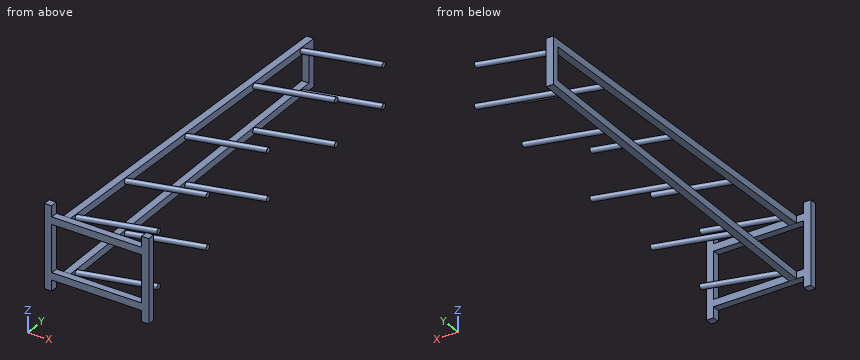
```python
from build123d import *

# Parameters (mm, degrees)
SKETCH1_W           = 25.4
SKETCH1_H           = 25.4
BOSS_EXTRUDE1_DEPTH = 292.1
SKETCH2_W           = 25.4
SKETCH2_H           = 25.4
BOSS_EXTRUDE2_DEPTH = 317.5
BOSS_EXTRUDE3_DEPTH = 25.4
SKETCH4_R           = 9.525
BOSS_EXTRUDE5_DEPTH = 254


with BuildPart() as part:
    # Sketch1 → Boss-Extrude1 (new body)
    with BuildSketch(Plane.XY):
        with Locations((12.7, 12.7)):
            Rectangle(SKETCH1_W, SKETCH1_H)
    boss_extrude1 = extrude(amount=BOSS_EXTRUDE1_DEPTH)

    # Sketch2 → Boss-Extrude2 (add)
    with BuildSketch(Plane(origin=(25.4, 0, 0), x_dir=(0, 0, -1), z_dir=(1, 0, 0))):
        with Locations((-241.3, 12.7)):
            Rectangle(SKETCH2_W, SKETCH2_H)
        with Locations((-50.8, 12.7)):
            Rectangle(SKETCH2_W, SKETCH2_H)
    extrude(amount=BOSS_EXTRUDE2_DEPTH)

    # Mirror1: Boss-Extrude1 across plane
    add(boss_extrude1.mirror(Plane(origin=(184.15, 0, 0), x_dir=(0, 0, 1), z_dir=(1, 0, 0))))

    # Sketch3 → Boss-Extrude3 (add)
    with BuildSketch(Plane.ZY.offset(-50.8)):
        Polygon((38.1, 25.4), (63.5, 1320.8), (88.904882268, 1320.8), (203.195117732, 1320.8), (228.6, 1320.8), (254, 25.4), (228.595117732, 25.4), (203.693156948, 1295.4), (88.406843052, 1295.4), (63.504882268, 25.4), align=None)
    extrude(amount=-BOSS_EXTRUDE3_DEPTH)

    # Sketch4 → Boss-Extrude5 (add, along a direction that is not the sketch's normal)
    with BuildSketch(Plane(origin=(76.2, 0, 0), x_dir=(0, 0, -1), z_dir=(1, 0, 0))):
        with Locations((-240.674544157, 57.298247998)):
            Circle(SKETCH4_R)
        with Locations((-235.530825048, 319.62792253)):
            Circle(SKETCH4_R)
        with Locations((-229.210655655, 641.956561596)):
            Circle(SKETCH4_R)
        with Locations((-217.142014813, 1257.457244551)):
            Circle(SKETCH4_R)
        with Locations((-222.108994477, 1004.141281654)):
            Circle(SKETCH4_R)
    boss_extrude5 = extrude(amount=BOSS_EXTRUDE5_DEPTH, dir=(0.9659258262890673, 0.2588190451025247, -2.638762530576281e-15))

    # Mirror2: Boss-Extrude5 across plane
    add(boss_extrude5.mirror(Plane.XY.offset(146.05)))


solid = part.part
```
Input: part model. Units: mm. Frame: model coordinates. Round coordinates to 2 decimals unless told otherwise and drop trailing zeros. Loops run counter-clockwise (first coordinate to the right, second up) from the corner with the lowest first, then second, coordinate; pieces in that order, holes last. Notation, with made-up numbers: (10, 9) - (15, 9) arc R19 ccw to (15, 17) - close; hole circle Ø4 at (-21, -16). An arc over 180 degrees is marked (long way). One line per item, written item: value. Start each with the question number.
(1) Section C-C, the plane x = 155.5. Count the separate pieces of the cut face and the enclosed holes in it, plus the area to 3 significant figures.
(2) Section B-B, the plane y = 792.5. Return loops of the section in (x, z), plus the area to 3 significant figures.
(3) Ray query, line 1 (Y direction, x = 298.5, z = 223.5); line 2 (X direction, y = 1221, z = 209); line 3 (Y direction, x = 286, z = 249). Return the intervals inside material, ascending. Write a range as [from, to].
(4) Section A-A, the plane z = 117. Return loops of the section in (x, y), plus the area to 3 significant figures.
(5) Contact query for flat-ended pins moving along their axis: P1, Ø15, axis at y = 121, z = 49, coming from the +X side; P2, Ø7.5, axis at x = 183, y = 7.5, coming from the +Z side; P3, Ø7.5, axis at x = 67, z = 159, coming from the +Y side. Output: stop coordinate, or through.
Results below:
1. separate pieces: 12
1. enclosed holes: 0
1. area: 4,140 mm^2
2. outline: (50.8, 53.14) - (76.2, 53.14) - (76.2, 78.55) - (50.8, 78.55) - close; (50.8, 213.55) - (76.2, 213.55) - (76.2, 238.96) - (50.8, 238.96) - close
2. area: 1,290 mm^2
3. line 1: [693.9, 709.14], [1054.28, 1073.13], [1309.93, 1324.11]
3. line 2: [50.8, 76.2]
3. line 3: [0, 25.4], [108.89, 118.14]
4. outline: (0, 0) - (25.4, 0) - (25.4, 25.4) - (0, 25.4) - close; (50.8, 1295.4) - (76.2, 1295.4) - (76.2, 1320.8) - (50.8, 1320.8) - close; (342.9, 0) - (368.3, 0) - (368.3, 25.4) - (342.9, 25.4) - close
4. area: 1,940 mm^2
5. P1: x = 321.55
5. P2: z = 254
5. P3: y = 1320.8
